from build123d import *

# Parameters (mm, degrees)
SKETCH1_W             = 50
SKETCH1_H             = 44
BOSS_EXTRUDE1_DEPTH   = 4
F_3_0MM_DOWEL_HOLE1_D = 3.2
SKETCH4_R             = 14
CUT_EXTRUDE1_DEPTH    = 4
F_3_0MM_DOWEL_HOLE2_D = 3


with BuildPart() as part:
    # Sketch1 → Boss-Extrude1 (new body)
    with BuildSketch(Plane.XY):
        with Locations((25, 22)):
            Rectangle(SKETCH1_W, SKETCH1_H)
    extrude(amount=BOSS_EXTRUDE1_DEPTH)

    # Ø3.0mm Dowel Hole1 (through all)
    with Locations(Plane.XY.offset(4)):
        with Locations((6.5, 34), (43.5, 34)):
            Hole(F_3_0MM_DOWEL_HOLE1_D / 2)

    # Sketch4 → Cut-Extrude1 (cut)
    with BuildSketch(Plane.XY.offset(4)):
        with Locations((25, 19)):
            Circle(SKETCH4_R)
    extrude(amount=-CUT_EXTRUDE1_DEPTH, mode=Mode.SUBTRACT)

    # Ø3.0mm Dowel Hole2 (through all)
    with Locations(Plane.XY.offset(4)):
        with Locations((12.5, 31.5), (25, 19), (37.5, 31.5), (37.5, 6.5), (12.5, 6.5)):
            Hole(F_3_0MM_DOWEL_HOLE2_D / 2)


solid = part.part
Work out the finished part from the listing and answer in its coordinate system (mm). Give positions to 0.01 mm unless a question says otherwise; leave off trailing zeros. Loops run counter-clockwise (first coordinate to the right, second up) from the corner with the lowest first, then second, coordinate; pieces in that order, holes last. Notation, with made-up numbers: (88.25, -8) -> (112.25, -8) arc R10 cw to (112.25, -2) -> close; hole circle Ø3 at (18, -25). An arc over 180 degrees is marked (long way). Use a Markdown table: item, result. Add a question column.
1. Section C-C on z = 2.25 is taken. Determine the outline of the cut face in (x, y).
2. Section B-B on x = 25 is taken. Determine the outline of the cut face in (y, z).
3. Section D-D on y = 6.5 is taken. Determine the outline of the cut face in (x, z).
4. Determine the mould class of faces 1 (the cylindrical face through (31.5, 6.6, 2)), 2 (the flat face through (19, 32, 4)), 3 (the flat face through (50, 22, 2)) for opening direction X: released by +X, released by -X, zero draft, split by the parting line, or undercut.
5. Section A-A on y = 19 is taken. Determine the outline of the cut face in (x, z).
6. Find the intervals of material crossed by probe 1 along X at (y, z) = (31, 0.7); probe 2 along Y at (x, z) = (37.5, 2.1); probe 3 along Y at (x, z) = (6.5, 1.1), in increasing order.
Results below:
| question | item | result |
|---|---|---|
| 1 | outline | (0, 0) -> (50, 0) -> (50, 44) -> (0, 44) -> close; hole circle Ø3.2 at (6.5, 34); hole circle Ø3 at (12.5, 6.5); hole circle Ø28 at (25, 19); hole circle Ø3 at (12.5, 31.5); hole circle Ø3 at (37.5, 6.5); hole circle Ø3 at (37.5, 31.5); hole circle Ø3.2 at (43.5, 34) |
| 2 | outline | (0, 0) -> (5, 0) -> (5, 4) -> (0, 4) -> close; (33, 0) -> (44, 0) -> (44, 4) -> (33, 4) -> close |
| 3 | outline | (0, 0) -> (11, 0) -> (11, 4) -> (0, 4) -> close; (14, 0) -> (18.7, 0) -> (18.7, 4) -> (14, 4) -> close; (31.3, 0) -> (36, 0) -> (36, 4) -> (31.3, 4) -> close; (39, 0) -> (50, 0) -> (50, 4) -> (39, 4) -> close |
| 4 | face 1 | undercut |
| 4 | face 2 | zero draft |
| 4 | face 3 | released by +X |
| 5 | outline | (0, 0) -> (11, 0) -> (11, 4) -> (0, 4) -> close; (39, 0) -> (50, 0) -> (50, 4) -> (39, 4) -> close |
| 6 | probe 1 | x = 0 to 11.09, 13.91 to 17.79, 32.21 to 36.09, 38.91 to 50 |
| 6 | probe 2 | y = 0 to 5, 8 to 12.7, 25.3 to 30, 33 to 44 |
| 6 | probe 3 | y = 0 to 32.4, 35.6 to 44 |
